Geometry: final body of the model. Coordinates: model frame, mm. Give positions to 0.01 mm unless a question says otherwise; leave off trailing zeros. Order: outer loops, then holes, each group sorted by start corner. A loop starts at its lowest first (then second) coordinate and runs counter-clockwise, first axis right, second up. Notation, with made-up numbers: (22, 10.5) -> (32, 10.5) arc R15 cw to (32, 21.5) -> close; hole circle Ø3 at (27.5, 67.5). An arc over 180 degrees is marked (long way). Answer in a Markdown table with one row per item. Add a question column.
Q1. Cut plane D-D on y = 29. Return the cut outline in (x, z).
Q2. Cut plane B-B on z = 0.2. Return the cut outline in (x, y) (3 decimals).
Q3. Cut plane A-A on x = 12.7. Return the cut outline in (y, z) (3 decimals).
Q4. Cut plane C-C on y = 21.5. Return the cut outline in (x, z), and give its area (3 significant figures).
Q5. Pull-direction query (X, two-part tool) for faces 1 (the face through (13, 17, 1.245)), 2 (the face through (12.54, 5.08, 0.61)), 3 (the face through (12.98, 33.65, 0.61)); classes: +X half, -X half, draft (parallel to the pull), parting line (faces both ways), or undercut.
Q6. Line query: line 1 along X through (y, z) = (21, 1.05); line 2 along X through (y, z) = (23.5, 0.85); line 3 along Y through (x, z) = (11, 0.3). Output: solid intervals per line, ascending. Write a range as from..to.
Q7. Contact query for flat-ended pins moving along their axis: P1, Ø12, axis at x = 16, y = 16.5, coming from the -Z side; P2, Ø5, axis at x = 12.7, y = 20.955, coming from the -Z side. Output: stop coordinate, or through.
from build123d import *

# Parameters (mm, degrees)
SKETCH1_R           = 3.175
BOSS_EXTRUDE1_DEPTH = 1.2446


with BuildPart() as part:
    # Sketch1 → Boss-Extrude1 (new body)
    with BuildSketch(Plane.XY):
        with BuildLine():
            Line((0, 0), (2.54, 0))
            ThreePointArc((2.54, 0), (12.7, 5.08), (22.86, 0))
            Line((22.86, 0), (25.4, 0))
            Line((25.4, 0), (25.4, 20.955))
            ThreePointArc((25.4, 20.955), (12.7, 33.655), (0, 20.955))
            Line((0, 20.955), (0, 0))
        make_face()
        with Locations((12.7, 20.955)):
            Circle(SKETCH1_R, mode=Mode.SUBTRACT)
    extrude(amount=BOSS_EXTRUDE1_DEPTH)


solid = part.part
Completed:
| question | item | result |
|---|---|---|
| 1 | outline | (2.87, 0) -> (22.53, 0) -> (22.53, 1.24) -> (2.87, 1.24) -> close |
| 2 | outline | (0, 0) -> (2.54, 0) arc R12.7 cw to (22.86, 0) -> (25.4, 0) -> (25.4, 20.955) arc R12.7 ccw to (0, 20.955) -> close; hole circle Ø6.35 at (12.7, 20.955) |
| 3 | outline | (5.08, 0) -> (17.78, 0) -> (17.78, 1.245) -> (5.08, 1.245) -> close; (24.13, 0) -> (33.655, 0) -> (33.655, 1.245) -> (24.13, 1.245) -> close |
| 4 | outline | (0.01, 0) -> (9.57, 0) -> (9.57, 1.24) -> (0.01, 1.24) -> close; (15.83, 0) -> (25.39, 0) -> (25.39, 1.24) -> (15.83, 1.24) -> close |
| 4 | area | 23.8 mm² |
| 5 | face 1 | draft |
| 5 | face 2 | undercut |
| 5 | face 3 | parting line |
| 6 | line 1 | x = 0..9.53, 15.87..25.4 |
| 6 | line 2 | x = 0.26..10.8, 14.6..25.14 |
| 6 | line 3 | y = 4.97..18.27, 23.64..33.54 |
| 7 | P1 | stops at z = 0 |
| 7 | P2 | passes through |
